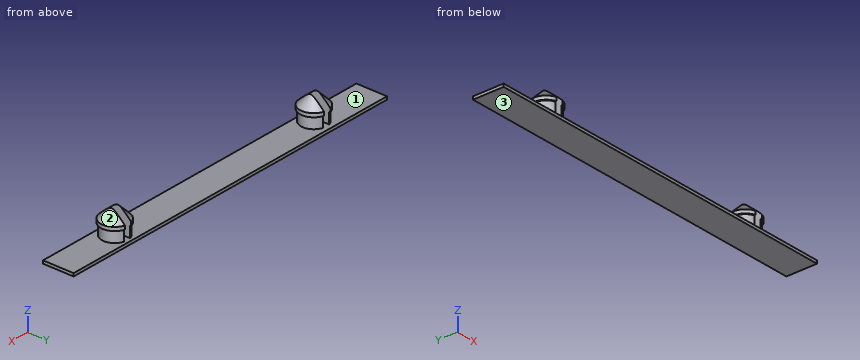
from build123d import *

# Parameters (mm, degrees)
SKICA2_W                 = 50
SKICA2_H                 = 4.2
P_IDAT_VYSUNUT_M2_DEPTH  = 0.4
SKICA3_R                 = 1.75
P_IDAT_VYSUNUT_M3_DEPTH  = 1.5
SKICA5_R                 = 1.9
P_IDAT_VYSUNUT_M5_DEPTH  = 2
ZKOSEN_2_SIZE            = 1.5
SKICA7_W                 = 1
SKICA7_H                 = 5
ODEBRAT_VYSUNUT_M1_DEPTH = 3.5


with BuildPart() as part:
    # Skica2 → Přidat vysunutím2 (new body)
    with BuildSketch(Plane.XY):
        Rectangle(SKICA2_W, SKICA2_H)
    extrude(amount=P_IDAT_VYSUNUT_M2_DEPTH)

    # Skica3 → Přidat vysunutím3 (add)
    with BuildSketch(Plane.XY.offset(0.4)):
        with Locations((-16, -0.2)):
            Circle(SKICA3_R)
        with Locations((16, 0)):
            Circle(SKICA3_R)
    extrude(amount=P_IDAT_VYSUNUT_M3_DEPTH)

    # Skica5 → Přidat vysunutím5 (add)
    with BuildSketch(Plane.XY.offset(1.9)):
        with Locations((-16, -0.2)):
            Circle(SKICA5_R)
        with Locations((16, 0)):
            Circle(SKICA5_R)
    extrude(amount=P_IDAT_VYSUNUT_M5_DEPTH)

    # Zkosení2
    zkosen_2_edges = [part.edges().sort_by_distance(p)[0] for p in [
        (-17.9, -0.2, 3.9),
        (14.1, 0, 3.9),
    ]]
    chamfer(zkosen_2_edges, length=ZKOSEN_2_SIZE)

    # Skica7 → Odebrat vysunutím1 (cut)
    with BuildSketch(Plane.XY.offset(3.9)):
        with Locations((-16, -0.2)):
            Rectangle(SKICA7_W, SKICA7_H)
        with Locations((16, 0)):
            Rectangle(SKICA7_W, SKICA7_H)
    extrude(amount=-ODEBRAT_VYSUNUT_M1_DEPTH, mode=Mode.SUBTRACT)


solid = part.part
Could you check a few things on this model? Use its own coordinates, in mm. Face numbers are marked on the shaded views. Coordinates: 2 decimals unless noted, no trailing zeros. Order: outer loops, then holes, each group sorted by start corner. A loop starts at its lowest first (then second) coordinate and runs counter-clockwise, first axis right, second up.
Q1. Suppose I cut it at B-B on x = 9. Please give me the cut outline in (y, z).
Q2. Thinking about a two-plate mould opening in X: for the marked faces 1, 2 and 3, which applies, released by +X, released by -X, zero draft, split by the parting line, or undercut?
Q3. Please list where these lines run through material, in increasing order: L1, parallel to X at y = -0.15, z = 1.5; L2, parallel to X at y = 0.55, z = 1.95; L3, parallel to Z at x = -19, y = -1.75.
Q4. Suppose I cut it at A-A on z = 1.4. Please give me the cut outline in (x, y), and give its area (3 significant figures).
Q5. Suppose I cut it at C-C on z = 3.35. Please give me the cut outline in (x, y).
Q6. Will these pins go through, and if not, where does the flat tip stop? pin 1 (1.5 mm diameter, centred on x = -10.5, y = 1, fed in from +Z); pin 2 (1 mm diameter, centred on y = -0.5, z = 1.5, fed in from -X).
Answer:
1. outline: (-2.1, 0) - (2.1, 0) - (2.1, 0.4) - (-2.1, 0.4) - close
2. face 1: undercut
2. face 2: released by +X
2. face 3: zero draft
3. L1: x = -17.75 to -16.5, -15.5 to -14.25, 14.26 to 15.5, 16.5 to 17.74
3. L2: x = -17.75 to -16.5, -15.5 to -14.25, 14.18 to 15.5, 16.5 to 17.82
3. L3: z = 0 to 0.4
4. outline: (-16.5, -1.88) - (-16.5, 1.48) arc R1.75 ccw to start; (-15.5, -1.88) arc R1.75 ccw to (-15.5, 1.48) - close; (15.5, -1.68) - (15.5, 1.68) arc R1.75 ccw to start; (16.5, -1.68) arc R1.75 ccw to (16.5, 1.68) - close
4. area: 12.3 mm2
5. outline: (-16.5, -1.01) - (-16.5, 0.61) arc R0.95 ccw to start; (-15.5, -1.01) arc R0.95 ccw to (-15.5, 0.61) - close; (15.5, -0.81) - (15.5, 0.81) arc R0.95 ccw to start; (16.5, -0.81) arc R0.95 ccw to (16.5, 0.81) - close
6. pin 1: stops at z = 0.4
6. pin 2: stops at x = -17.9
